from build123d import *

# Parameters (mm, degrees)
SKETCH_1_W      = 500
SKETCH_1_H      = 400
EXTRUDE_1_DEPTH = 20
SKETCH_2_W      = 40
SKETCH_2_H      = 40
EXTRUDE_2_DEPTH = 280
EXTRUDE_3_DEPTH = 40
EXTRUDE_START   = -360
EXTRUDE_4_DEPTH = 40
EXTRUDE_5_DEPTH = 40
EXTRUDE_START_2 = -460
EXTRUDE_6_DEPTH = 40


with BuildPart() as part:
    # 草图1 → 凸台-拉伸1 (new body)
    with BuildSketch(Plane.XY):
        Rectangle(SKETCH_1_W, SKETCH_1_H)
    extrude(amount=EXTRUDE_1_DEPTH)

    # 草图2 → 凸台-拉伸2 (add)
    with BuildSketch(Plane(origin=(0, 0, 0), x_dir=(-1, 0, 0), z_dir=(0, 0, -1))):
        with Locations((-230, 180)):
            Rectangle(SKETCH_2_W, SKETCH_2_H)
        with Locations((230, 180)):
            Rectangle(SKETCH_2_W, SKETCH_2_H)
        with Locations((230, -180)):
            Rectangle(SKETCH_2_W, SKETCH_2_H)
        with Locations((-230, -180)):
            Rectangle(SKETCH_2_W, SKETCH_2_H)
    extrude(amount=EXTRUDE_2_DEPTH)

    # 草图3 → 凸台-拉伸3 (add)
    with BuildSketch(Plane(origin=(0, 200, 0), x_dir=(1, 0, 0), z_dir=(0, 1, 0))):
        Polygon((-210, 160), (-50, 0), (-106.568542495, 0), (-210, 103.431457505), align=None)
        Polygon((106.568542495, 0), (210, 103.431457505), (210, 160), (50, 0), align=None)
    extrude(amount=-EXTRUDE_3_DEPTH)

    # 草图3<3> → 凸台-拉伸4 (add)
    with BuildSketch(Plane(origin=(0, 200, 0), x_dir=(1, 0, 0), z_dir=(0, 1, 0)).offset(EXTRUDE_START)):
        Polygon((-210, 160), (-50, 0), (-106.568542495, 0), (-210, 103.431457505), align=None)
        Polygon((106.568542495, 0), (210, 103.431457505), (210, 160), (50, 0), align=None)
    extrude(amount=-EXTRUDE_4_DEPTH)

    # 草图4 → 凸台-拉伸5 (add)
    with BuildSketch(Plane(origin=(250, 0, 0), x_dir=(0, 0, -1), z_dir=(1, 0, 0))):
        Polygon((0, 50), (110, 160), (53.431457505, 160), (0, 106.568542495), align=None)
        Polygon((53.431457505, -160), (0, -106.568542495), (0, -50), (110, -160), align=None)
    extrude(amount=-EXTRUDE_5_DEPTH)

    # 草图4<2> → 凸台-拉伸6 (add)
    with BuildSketch(Plane(origin=(250, 0, 0), x_dir=(0, 0, -1), z_dir=(1, 0, 0)).offset(EXTRUDE_START_2)):
        Polygon((0, 50), (110, 160), (53.431457505, 160), (0, 106.568542495), align=None)
        Polygon((53.431457505, -160), (0, -106.568542495), (0, -50), (110, -160), align=None)
    extrude(amount=-EXTRUDE_6_DEPTH)


solid = part.part
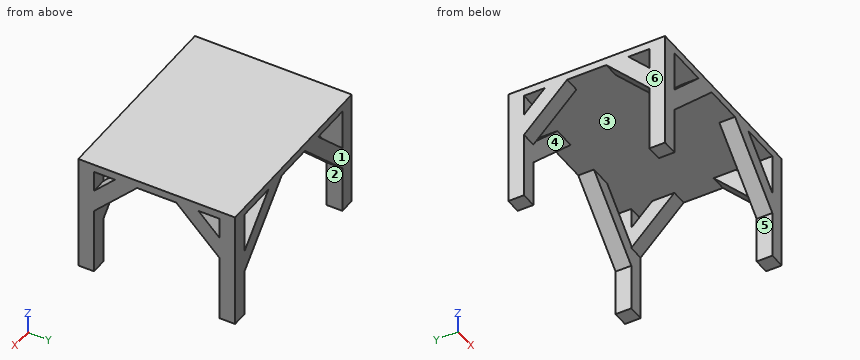
Part model, mm, in its own coordinate system. Face numbers are marked on the shaded views. A direction names the side the tool comes from. Coordinates: 2 decimals unless noted, no trailing zeros. Order: outer loops, then holes, each group sorted by start corner. A loop starts at its lowest first (then second) coordinate and runs counter-clockwise, first axis right, second up. Notation, with made-up numbers: (52.25, -7.75) - (63.25, -7.75) arc R25 cw to (63.25, 28.25) - close; hole circle Ø6 at (58, 89). An arc over 180 degrees is marked (long way). Use CSV: the item, a comma, the result in double quotes.
Item 1: Drop a flat-ended pin along its axis: P1, Ø10, axis at x = 145, z = -109, coming from the +Y side. Give the stop position or say it passes through.
Solved:
P1,"passes through"
Item 2: Saw through at D-D on z = -209. Give the cut face in (x, y).
Solved:
outline,"(-250, -200) - (-210, -200) - (-210, -160) - (-250, -160) - close; (-250, 160) - (-210, 160) - (-210, 200) - (-250, 200) - close; (210, -200) - (250, -200) - (250, -160) - (210, -160) - close; (210, 160) - (250, 160) - (250, 200) - (210, 200) - close"
Item 3: 3-axis set-ups, long thin cutter, end or side, ignore diameter. For the marked faces 4, 5 and 6: which of +Z, -Z, +X, -X, +Y, -Y reach the whole face in a straight line?
Solved:
face 4,"-Z"
face 5,"-Z, +Y, -Y"
face 6,"+Z, -Z, -X, +Y, -Y"
Item 4: Saw through at C-C on y = 88. Give the cut face in (x, z), and give its area (3 significant figures).
Solved:
outline,"(-250, -38) - (-210, -38) - (-210, 0) - (210, 0) - (210, -38) - (250, -38) - (250, 20) - (-250, 20) - close"
area,"13,000 mm²"
Item 5: Saw through at B-B on y = 140. Give the cut face in (x, z), and give its area (3 significant figures).
Solved:
outline,"(-250, -90) - (-210, -90) - (-210, -33.43) - (-250, -33.43) - close; (-250, 0) - (250, 0) - (250, 20) - (-250, 20) - close; (210, -90) - (250, -90) - (250, -33.43) - (210, -33.43) - close"
area,"14,500 mm²"
Item 6: Mould opens along Y. For the marked faces 1, 2 and 3 say: +Y half, -Y half, draft (parallel to the pull), parting line (faces both ways), or undercut.
Solved:
face 1,"+Y half"
face 2,"draft"
face 3,"undercut"
Item 7: Probe probe 1 along Y at (x, z) = (212, -158); probe 2 along Z at (x, y) = (-116.5, 6.5); probe 3 along Y at (x, z) = (220, -4). List the from-to ranges inside material, lowest first.
Solved:
probe 1,"y = -200 to -160, 160 to 200"
probe 2,"z = 0 to 20"
probe 3,"y = -200 to -160, -110.57 to -54, 54 to 110.57, 160 to 200"
Item 8: Saw through at A-A on z = -134.5. Give the cut face in (x, y).
Solved:
outline,"(-250, -200) - (-184.5, -200) - (-184.5, -160) - (-250, -160) - close; (-250, 160) - (-184.5, 160) - (-184.5, 200) - (-250, 200) - close; (184.5, -200) - (250, -200) - (250, -160) - (184.5, -160) - close; (184.5, 160) - (250, 160) - (250, 200) - (184.5, 200) - close"
